from build123d import *

# Parameters (mm, degrees)
F0_W     = 63.754
F0_H     = 38.354
F1_DEPTH = 6.5024
F2_W     = 51.054
F2_H     = 38.354
F3_DEPTH = 18.796
F4_W     = 38.4032912552
F4_H     = 8.6150002171
F5_DEPTH = 25.4
F7_DEPTH = 18.797


with BuildPart() as f1:
    # F0 (on Top) → F1 (new body)
    with BuildSketch(Plane.XY):
        with Locations((0, -0.0474722673)):
            Rectangle(F0_W, F0_H)
    extrude(amount=F1_DEPTH)

    # F2 (on Top) → F3 (join)
    with BuildSketch(Plane.XY):
        with Locations((0, 0.243213877)):
            Rectangle(F2_W, F2_H)
    extrude(amount=F3_DEPTH)

    # F4 (on face) → F5 (cut)
    with BuildSketch(Plane.XY.offset(18.796)):
        with Locations((0.0579152256, -14.6262860144)):
            Rectangle(F4_W, F4_H)
    extrude(amount=-F5_DEPTH, mode=Mode.SUBTRACT)

    # F6 (on face) → F7 (cut, through all)
    with BuildSketch(Plane.XY.offset(18.796)):
        with BuildLine():
            ThreePointArc((11.0276596023, 18.7562172295), (11.0228780842, 19.0883531968), (11.0085374932, 19.420213877))
            Line((11.0085374932, 19.420213877), (-12.0289784785, 19.420213877))
            ThreePointArc((-12.0289784785, 19.420213877), (-0.8423564599, 7.2231186526), (11.0276596023, 18.7562172295))
        make_face()
    extrude(amount=-F7_DEPTH, mode=Mode.SUBTRACT)


solid = f1.part
Geometry check sheet. Reference: the model listing, model coordinates, mm. A direction names the side the tool comes from. Give positions to 0.01 mm unless a question says otherwise; leave off trailing zeros. Order: outer loops, then holes, each group sorted by start corner. A loop starts at its lowest first (then second) coordinate and runs counter-clockwise, first axis right, second up.
1) Cross-section at A-A (z = 4). Record the boundary of the cut face in (x, y).
Results are:
outline: (-31.88, -19.22) - (31.88, -19.22) - (31.88, 19.13) - (25.53, 19.13) - (25.53, 19.42) - (11.01, 19.42) arc R11.54 cw (long way) to (-12.03, 19.42) - (-25.53, 19.42) - (-25.53, 19.13) - (-31.88, 19.13) - close; hole (-19.14, -18.93) - (19.26, -18.93) - (19.26, -10.32) - (-19.14, -10.32) - close
2) Material ranges on probe 1 along X at (y, z) = (-16, 3.5); probe 2 along X at (y, z) = (-11.5, 7.5); probe 3 along Z at (x, y) = (27, 0.5), recorded low to high.
Results are:
probe 1: x = -31.88 to -19.14, 19.26 to 31.88
probe 2: x = -25.53 to -19.14, 19.26 to 25.53
probe 3: z = 0 to 6.5
3) Cross-section at C-C (y = -3.5). Record the boundary of the cut face in (x, z).
Results are:
outline: (-31.88, 0) - (31.88, 0) - (31.88, 6.5) - (25.53, 6.5) - (25.53, 18.8) - (-25.53, 18.8) - (-25.53, 6.5) - (-31.88, 6.5) - close
4) Gauge pin test, flat ends, axial feed: pin 1 (1.5 mm diameter, centred on x = -11, y = -5, fed in from -Z); pin 2 (4 mm diameter, centred on x = -24, z = 12.5, fed in from -Y); pin 3 (6 mm diameter, centred on y = 3, z = 16, fed in from +X); pin 4 (3 mm diameter, centred on x = 28, z = 1.5, fed in from +Y). Record the tip position at first contact, or that the pin passes through.
Results are:
pin 1: stops at z = 0
pin 2: stops at y = -18.93
pin 3: stops at x = 25.53
pin 4: stops at y = 19.13
5) Cross-section at B-B (x = 13.5). Record the boundary of the cut face in (y, z).
Results are:
outline: (-19.22, 0) - (-18.93, 0) - (-18.93, 6.5) - (-19.22, 6.5) - close; (-10.32, 0) - (19.42, 0) - (19.42, 18.8) - (-10.32, 18.8) - close
6) Cross-section at D-D (y = 14). Record the boundary of the cut face in (x, z), then the cut area to 3 significant figures.
Results are:
outline: (-31.88, 0) - (-11.02, 0) - (-11.02, 18.8) - (-25.53, 18.8) - (-25.53, 6.5) - (-31.88, 6.5) - close; (10, 0) - (31.88, 0) - (31.88, 6.5) - (25.53, 6.5) - (25.53, 18.8) - (10, 18.8) - close
area: 647 mm2
7) Tool access check on faces 4 (the flat face through (-29, 19.13, 3)), 5 (the flat face through (-22, -18.934, 13)), 6 (the flat face through (19.26, -15, 10)), 7 (the flat face through (29, 19.13, 3)). Record the directions out of +Z, -Z, +X, -X, +Y, -Y that give a thin tool (end or side, any length) a straight path to the whole face; none if there is none.
Results are:
face 4: +Z, -Z, -X, +Y
face 5: +Z, +X, -X, -Y
face 6: +Z, -Z
face 7: +Z, -Z, +X, +Y
8) Draft check along X on faces 1 (the flat face through (0, -18.934, 3)), 2 (the flat face through (22, -18.934, 13)), 3 (the flat face through (31.877, 0, 3)). Enter one of: released by +X, released by -X, zero draft, split by the parting line, or undercut.
Results are:
face 1: undercut
face 2: zero draft
face 3: released by +X
